```python
from build123d import *

# Parameters (mm, degrees)
SKETCH1_W           = 50.8
SKETCH1_H           = 203.2
BOSS_EXTRUDE2_DEPTH = 38.1
SKETCH2_R           = 9.525
CUT_EXTRUDE1_DEPTH  = 38.1
SKETCH3_R           = 9.525
CUT_EXTRUDE2_DEPTH  = 38.1
SKETCH4_W           = 254
SKETCH4_H           = 254.028971003
CUT_EXTRUDE3_DEPTH  = 7.62
CHAMFER1_SIZE       = 7.62


with BuildPart() as part:
    # Sketch1 → Boss-Extrude2 (new body)
    with BuildSketch(Plane(origin=(0, 0, 0), x_dir=(1, 0, 0), z_dir=(0, 1, 0))):
        Polygon((0, 0), (0, 25.4), (-50.8, 25.4), (-101.6, 25.4), (-152.4, 25.4), (-203.2, 25.4), (-203.2, 228.6), (-228.6, 228.6), (-228.6, 0), align=None)
        with Locations((-127, 127)):
            Rectangle(SKETCH1_W, SKETCH1_H)
        with Locations((-25.4, 127)):
            Rectangle(SKETCH1_W, SKETCH1_H)
    extrude(amount=BOSS_EXTRUDE2_DEPTH)

    # Sketch2 → Cut-Extrude1 (cut)
    with BuildSketch(Plane(origin=(0, 0, -228.6), x_dir=(-1, 0, 0), z_dir=(0, 0, -1))):
        with Locations((215.9, 19.05)):
            Circle(SKETCH2_R)
    extrude(amount=-CUT_EXTRUDE1_DEPTH, mode=Mode.SUBTRACT)

    # Sketch3 → Cut-Extrude2 (cut)
    with BuildSketch(Plane(origin=(0, 0, 0), x_dir=(0, 0, -1), z_dir=(1, 0, 0))):
        with Locations((12.728971003, 19.05)):
            Circle(SKETCH3_R)
    extrude(amount=-CUT_EXTRUDE2_DEPTH, mode=Mode.SUBTRACT)

    # Sketch4 → Cut-Extrude3 (cut)
    with BuildSketch(Plane(origin=(0, 38.1, 0), x_dir=(1, 0, 0), z_dir=(0, 1, 0))):
        with Locations((50.8, 152.414485501)):
            Rectangle(SKETCH4_W, SKETCH4_H)
    extrude(amount=-CUT_EXTRUDE3_DEPTH, mode=Mode.SUBTRACT)

    # Chamfer1
    chamfer1_edges = [part.edges().sort_by_distance(p)[0] for p in [
        (-114.3, 0, 0),
        (-228.6, 0, -114.3),
        (-228.6, 38.1, -114.3),
        (-114.3, 38.1, 0),
    ]]
    chamfer(chamfer1_edges, length=CHAMFER1_SIZE)


solid = part.part
```
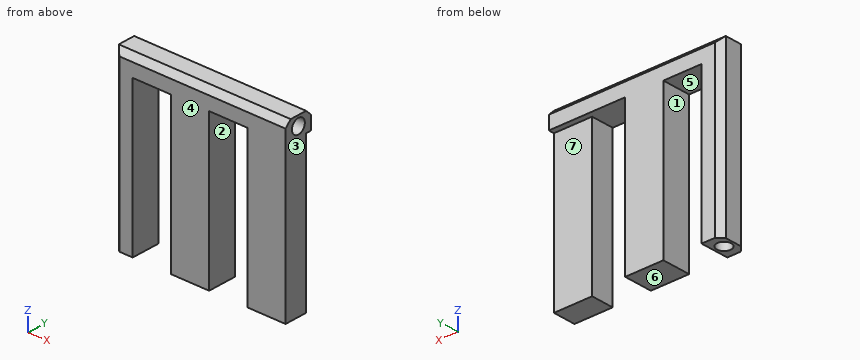
The model under review builds one solid part; all positions refer to its coordinate system, in mm. Face numbers are marked on the shaded views. A direction names the side the tool comes from. Round coordinates to 2 decimals unless told otherwise and drop trailing zeros. Loops run counter-clockwise (first coordinate to the right, second up) from the corner with the lowest first, then second, coordinate; pieces in that order, holes last.
Item 1: Take a section at A-A (z = -106.5). Write out the cut boundary in (x, y).
Determined:
outline: (-228.6, 7.62) - (-220.98, 0) - (-203.2, 0) - (-203.2, 38.1) - (-220.98, 38.1) - (-228.6, 30.48) - close; (-152.4, 0) - (-101.6, 0) - (-101.6, 38.1) - (-152.4, 38.1) - close; (-50.8, 0) - (0, 0) - (0, 30.48) - (-50.8, 30.48) - close
Item 2: Mouldability with a two-part tool opening along X and no side actions: class the marked faces 1, 2, 3 and 4 as released by +X, released by -X, zero draft, split by the parting line, or undercut.
Determined:
face 1: undercut
face 2: undercut
face 3: released by +X
face 4: zero draft
Item 3: For line 1 (X direction, y = 26, z = -161.5); line 2 (X direction, y = 6, z = -113); line 3 (X direction, y = 19, z = -212), list the stretches that pass through material, from the lowest coordinate up.
Determined:
line 1: x = -228.6 to -203.2, -152.4 to -101.6, -50.8 to 0
line 2: x = -226.98 to -203.2, -152.4 to -101.6, -50.8 to 0
line 3: x = -228.6 to -225.42, -206.38 to -203.2, -152.4 to -101.6, -50.8 to 0
Item 4: For the marked faces 5, 6 and 7, list the 3-axis set-ups (+Z, -Z, +X, -X, +Y, -Y) from which the entire face can be reached by the end or side of a thin tool; tool diameter is ignored.
Determined:
face 5: -Z, +Y, -Y
face 6: -Z, +X, -X, +Y, -Y
face 7: -Z, +X, +Y
Item 5: Clearance check with flat-ended pins moving along their axes: pin 1 Ø1.5 at (y, z) = (33, -36.5) entering from +X; pin 2 Ø11.5 at (x, y) = (-172.5, 27.5) entering from -Z; pin 3 Ø8 at (x, z) = (-31.5, -148.5) entering from +Y. State where each tip first meets the part, or that it passes through.
Determined:
pin 1: stops at x = -101.6
pin 2: stops at z = -25.4
pin 3: stops at y = 30.48
Item 6: Take a section at D-D (x = -215.9). Write out the cut boundary in (y, z) (3 decimals).
Determined:
outline: (0, -228.6) - (9.525, -228.6) - (9.525, -190.5) - (28.575, -190.5) - (28.575, -228.6) - (38.1, -228.6) - (38.1, -7.62) - (30.48, 0) - (7.62, 0) - (0, -7.62) - close
Item 7: Take a section at C-C (y = 19.05). Write out the cut boundary in (x, z) (3 decimals), then the cut area to 3 significant figures.
Determined:
outline: (-228.6, -228.6) - (-225.425, -228.6) - (-225.425, -190.5) - (-206.375, -190.5) - (-206.375, -228.6) - (-203.2, -228.6) - (-203.2, -25.4) - (-152.4, -25.4) - (-152.4, -228.6) - (-101.6, -228.6) - (-101.6, -25.4) - (-50.8, -25.4) - (-50.8, -228.6) - (0, -228.6) - (0, -22.254) - (-38.1, -22.254) - (-38.1, -3.204) - (0, -3.204) - (0, 0) - (-228.6, 0) - close
area: 30,200 mm2
Item 8: Take a section at B-B (x = -23.5). Write out the cut boundary in (y, z) (3 decimals), then the cut area to 3 significant figures.
Determined:
outline: (0, -228.6) - (30.48, -228.6) - (30.48, -25.4) - (38.1, -25.4) - (38.1, -7.62) - (30.48, 0) - (7.62, 0) - (0, -7.62) - close; hole circle Ø19.05 at (19.05, -12.729)
area: 6,820 mm2
